Input: part model. Units: mm. Frame: model coordinates. A direction names the side the tool comes from. Give positions to 0.01 mm unless a question says otherwise; leave off trailing zeros. Order: outer loops, then holes, each group sorted by start corner. A loop starts at its lowest first (then second) coordinate and runs counter-clockwise, first axis right, second up. Notation, with made-up numbers: (61.25, -22.5) - (104.25, -22.5) arc R22 ccw to (104.25, -1.5) - close; hole circle Ø9 at (9, 70.25). An arc over 180 degrees is marked (long way). Answer in a Markdown table with one row per item. Add a question column.
1. Access query for faces 1 (the face through (1, 0, 2.54)), 2 (the face through (-0.096, -0.434, -1.19)), 3 (the face through (0, 1.27, 1)). Directions: +Z, -Z, +X, -X, +Y, -Y. A direction counts if a zero-diameter tool reaches every point of the face in a straight line with its end or side. Return the directions, or none.
2. Section query D-D on x = -0.95. Return loops of the section in (y, z) (3 decimals).
3. Section query C-C on z = -1. Return loops of the section in (x, y).
4. Contact query for flat-ended pins moving along their axis: pin 1 (1 mm diameter, centred on x = 0, y = 0.5, fed in from +Z); pin 2 (1.5 mm diameter, centred on y = 0, z = 3.5, fed in from -X). Output: stop coordinate, or through.
5. Ray query, line 1 (Z direction, x = 0.9, y = 0.95); line 2 (Y direction, x = 0, z = 3.25); line 3 (X direction, y = 0.3, z = -0.5). Return the intervals inside material, ascending. Write a range as [from, to].
6. Section query A-A on x = 0. Return loops of the section in (y, z).
Autodesk Inventor part; units mm, degrees
ref_plane "YZ Plane" through (0, 0, 0) normal (1, 0, 0) x (0, 1, 0)
ref_plane "XZ Plane" through (0, 0, 0) normal (0, 1, 0) x (-1, 0, 0)
ref_plane "XY Plane" through (0, 0, 0) normal (0, 0, 1) x (1, 0, 0)
sketch "Sketch1" plane through (0, 0, 0) normal (0, 0, 1) x (1, 0, 0)
  circle A0 centre (0, 0) radius 0.4445
  dimension "d0" = 0.889
extrude "Extrusion1" add sketch "Sketch1" along normal blind 8.509 and the other way blind 2.54
chamfer "Chamfer1" distance 0.127 angle 45 2 edges at (-0.4445, 0, 8.509) (-0.4445, 0, -2.54)
sketch "Sketch2" plane through (0, 0, 0) normal (0, 0, 1) x (1, 0, 0)
  line L0 (-1.27, 1.27) -> (1.27, 1.27)
  line L1 (1.27, 1.27) -> (1.27, -1.27)
  line L2 (1.27, -1.27) -> (-1.27, -1.27)
  line L3 (-1.27, -1.27) -> (-1.27, 1.27)
  point P0 (0, 0)
  point P1 (1.27, 0)
  point P2 (0, 1.27)
  dimension "d8" = 2.54
  dimension "d9" = 2.54
extrude "Extrusion2" add sketch "Sketch2" along normal blind 2.54
chamfer "Chamfer2" distance 0.635 angle 45 4 edges at (1.27, 1.27, 1.27) (-1.27, 1.27, 1.27) (1.27, -1.27, 1.27) (-1.27, -1.27, 1.27)
properties part number "Pin"
Answer:
| question | item | result |
|---|---|---|
| 1 | face 1 | +Z |
| 1 | face 2 | -Z |
| 1 | face 3 | +Z, -Z, +X, -X, +Y |
| 2 | outline | (-0.955, 0) - (0.955, 0) - (0.955, 2.54) - (-0.955, 2.54) - close |
| 3 | outline | circle Ø0.89 at (0, 0) |
| 4 | pin 1 | stops at z = 8.51 |
| 4 | pin 2 | stops at x = -0.44 |
| 5 | line 1 | z = [0, 2.54] |
| 5 | line 2 | y = [-0.44, 0.44] |
| 5 | line 3 | x = [-0.33, 0.33] |
| 6 | outline | (-1.27, 0) - (-0.44, 0) - (-0.44, -2.41) - (-0.32, -2.54) - (0.32, -2.54) - (0.44, -2.41) - (0.44, 0) - (1.27, 0) - (1.27, 2.54) - (0.44, 2.54) - (0.44, 8.38) - (0.32, 8.51) - (-0.32, 8.51) - (-0.44, 8.38) - (-0.44, 2.54) - (-1.27, 2.54) - close |
